```python
from build123d import *

# Parameters (mm, degrees)
BOSS_EXTRUDE1_DEPTH = 45
SKETCH2_R           = 2.25
CUT_EXTRUDE1_DEPTH  = 55.472470111


with BuildPart() as part:
    # Sketch1 → Boss-Extrude1 (new body)
    with BuildSketch(Plane.XY):
        Polygon((-12.5, -2.5), (-12.5, -4), (12.5, -4), (12.5, -2.5), (30, -2.5), (30, 2.5), (-30, 2.5), (-30, -2.5), align=None)
    extrude(amount=BOSS_EXTRUDE1_DEPTH)

    # Sketch2 → Cut-Extrude1 (cut, through all)
    with BuildSketch(Plane(origin=(0, 2.5, 0), x_dir=(1, 0, 0), z_dir=(0, 1, 0))):
        with Locations(Location((-21.25, -7.5, 0), (0, 0, 180))):
            Circle(SKETCH2_R)
        with Locations(Location((-21.25, -22.5, 0), (0, 0, 180))):
            Circle(SKETCH2_R)
        with Locations(Location((-21.25, -37.5, 0), (0, 0, 180))):
            Circle(SKETCH2_R)
        with Locations(Location((21.25, -37.5, 0), (0, 0, 180))):
            Circle(SKETCH2_R)
        with Locations(Location((21.25, -22.5, 0), (0, 0, 180))):
            Circle(SKETCH2_R)
        with Locations(Location((21.25, -7.5, 0), (0, 0, 180))):
            Circle(SKETCH2_R)
    extrude(amount=-CUT_EXTRUDE1_DEPTH, mode=Mode.SUBTRACT)


solid = part.part
```
Verification items for the finished model (mm, model axes). A direction names the side the tool comes from. Coordinates: 2 decimals unless noted, no trailing zeros. Loops run counter-clockwise (first coordinate to the right, second up) from the corner with the lowest first, then second, coordinate; pieces in that order, holes last. Notation, with made-up numbers: (-5, 88) - (36, 88) arc R15 cw to (36, 113) - close; hole circle Ø9 at (85.25, 18.25). An arc over 180 degrees is marked (long way). Return JSON: item names as keys, results as strings.
1. Thickness scan on L1, parallel to Z at x = -21.25, y = 1.1; L2, parallel to X at y = -2, z = 8.5; L3, parallel to Y at x = 13.5, z = 14. Record the ranges inside material, lowest first.
Established:
{"L1": "z = 0 to 5.25, 9.75 to 20.25, 24.75 to 35.25, 39.75 to 45", "L2": "x = -30 to -23.27, -19.23 to 19.23, 23.27 to 30", "L3": "y = -2.5 to 2.5"}
2. Section check B-B, the plane x = -21.25. Record the boundary of the cut face in (y, z).
Established:
{"outline": "(-2.5, 0) - (2.5, 0) - (2.5, 5.25) - (-2.5, 5.25) - close; (-2.5, 9.75) - (2.5, 9.75) - (2.5, 20.25) - (-2.5, 20.25) - close; (-2.5, 24.75) - (2.5, 24.75) - (2.5, 35.25) - (-2.5, 35.25) - close; (-2.5, 39.75) - (2.5, 39.75) - (2.5, 45) - (-2.5, 45) - close"}
3. Tool access check on faces 1 (the flat face through (0, 0, 0)), 2 (the flat face through (-12.5, -3, 22)), 3 (the flat face through (25, -2.5, 22)). Record the directions out of +Z, -Z, +X, -X, +Y, -Y that give a thin tool (end or side, any length) a straight path to the whole face; none if there is none.
Established:
{"face 1": "-Z, +X, -X, +Y, -Y", "face 2": "+Z, -Z, -X, -Y", "face 3": "+Z, -Z, +X, -Y"}
4. Section check D-D, the plane z = 4. Record the boundary of the cut face in (x, y).
Established:
{"outline": "(-30, -2.5) - (-12.5, -2.5) - (-12.5, -4) - (12.5, -4) - (12.5, -2.5) - (30, -2.5) - (30, 2.5) - (-30, 2.5) - close"}
5. Section check C-C, the plane y = 0. Record the boundary of the cut face in (x, z), then the cut area to 3 significant figures.
Established:
{"outline": "(-30, 0) - (30, 0) - (30, 45) - (-30, 45) - close; hole circle Ø4.5 at (-21.25, 7.5); hole circle Ø4.5 at (-21.25, 22.5); hole circle Ø4.5 at (-21.25, 37.5); hole circle Ø4.5 at (21.25, 7.5); hole circle Ø4.5 at (21.25, 22.5); hole circle Ø4.5 at (21.25, 37.5)", "area": "2,600 mm2"}
6. Section check A-A, the plane z = 37.5. Record the boundary of the cut face in (x, y), then the cut area to 4 significant figures.
Established:
{"outline": "(-30, -2.5) - (-23.5, -2.5) - (-23.5, 2.5) - (-30, 2.5) - close; (-19, -2.5) - (-12.5, -2.5) - (-12.5, -4) - (12.5, -4) - (12.5, -2.5) - (19, -2.5) - (19, 2.5) - (-19, 2.5) - close; (23.5, -2.5) - (30, -2.5) - (30, 2.5) - (23.5, 2.5) - close", "area": "292.5 mm2"}
7. Mould release check, pull along Z, two halves, no side actions. Record for faces 4 (the flat face through (-17, -2.5, 22)), 5 (the cylindrical face through (19.104, 0.035, 8.176)), 6 (the flat face through (0, 0, 45)), 7 (the cylindrical face through (20.212, 0.035, 20.504)): +Z half, -Z half, draft (parallel to the pull), parting line (faces both ways), or undercut.
Established:
{"face 4": "draft", "face 5": "undercut", "face 6": "+Z half", "face 7": "undercut"}
8. Go/stop test with flat-tipped pins: pin 1 (2.5 mm diameter, centred on x = -21.25, z = 22.5, fed in from +Y); pin 2 (1.2 mm diameter, centred on y = -3, z = 23, fed in from +X); pin 3 (14 mm diameter, centred on x = 20.5, z = 17, fed in from -Y); pin 4 (1.6 mm diameter, centred on y = -3.5, z = 20.5, fed in from -X). Record where each tip stops, or that it passes through.
Established:
{"pin 1": "passes through", "pin 2": "stops at x = 30", "pin 3": "stops at y = -2.5", "pin 4": "stops at x = -12.5"}
